from build123d import *

# Parameters (mm, degrees)
BOX008_W                  = 10
BOX008_H                  = 10
BOX008_DEPTH              = 10
BOX008_PLACEMENT_ANGLE    = 45
BOX010_W                  = 10
BOX010_H                  = 10
BOX010_DEPTH              = 10
BOX010_PLACEMENT_ANGLE    = 45
BOX011_W                  = 10
BOX011_H                  = 10
BOX011_DEPTH              = 10
BOX011_PLACEMENT_ANGLE    = 45
BOX009_W                  = 10
BOX009_H                  = 10
BOX009_DEPTH              = 10
BOX009_PLACEMENT_ANGLE    = 45
CYLINDER002_R             = 20
CYLINDER002_DEPTH         = 105
CYLINDER003_R             = 20
CYLINDER003_DEPTH         = 105
CYLINDER001_R             = 3
CYLINDER001_DEPTH         = 105
BOX004_W                  = 105
BOX004_H                  = 105
BOX004_DEPTH              = 3
BOX004_PLACEMENT_ANGLE    = 60
BOX005_W                  = 105
BOX005_H                  = 105
BOX005_DEPTH              = 3
BOX005_PLACEMENT_ANGLE    = 60
BOX006_W                  = 105
BOX006_H                  = 105
BOX006_DEPTH              = 3
FUSION001_PLACEMENT_ANGLE = 90
CYLINDER_R                = 3
CYLINDER_DEPTH            = 105
BOX003_W                  = 105
BOX003_H                  = 105
BOX003_DEPTH              = 3
BOX003_PLACEMENT_ANGLE    = 300
BOX002_W                  = 105
BOX002_H                  = 105
BOX002_DEPTH              = 3
BOX002_PLACEMENT_ANGLE    = 60
BOX001_W                  = 105
BOX001_H                  = 105
BOX001_DEPTH              = 3
CYLINDER005_R             = 2
CYLINDER005_DEPTH         = 10
CYLINDER004_R             = 2
CYLINDER004_DEPTH         = 10
BOX007_W                  = 4
BOX007_H                  = 4
BOX007_DEPTH              = 10
FUSION004_PLACEMENT_ANGLE = 90
BOX_W                     = 12
BOX_H                     = 4
BOX_DEPTH                 = 12
FILLET_R                  = 3


with BuildPart() as cube008:
    # Box008 → Box008 (new body)
    with BuildSketch(Plane.XY):
        with Locations((5, 5)):
            Rectangle(BOX008_W, BOX008_H)
    extrude(amount=BOX008_DEPTH)


with BuildPart() as cube008_1:
    # Box008 placement: moved
    add(cube008.part.moved(Location((-3, -11, 0))).rotate(Axis((-3, -11, 0), (0, 0, 1)), BOX008_PLACEMENT_ANGLE))


with BuildPart() as cube010:
    # Box010 → Box010 (new body)
    with BuildSketch(Plane.XY):
        with Locations((5, 5)):
            Rectangle(BOX010_W, BOX010_H)
    extrude(amount=BOX010_DEPTH)


with BuildPart() as cube010_1:
    # Box010 placement: moved
    add(cube010.part.moved(Location((108.2, -11, 0))).rotate(Axis((108.2, -11, 0), (0, 0, 1)), BOX010_PLACEMENT_ANGLE))


with BuildPart() as cube011:
    # Box011 → Box011 (new body)
    with BuildSketch(Plane.XY):
        with Locations((5, 5)):
            Rectangle(BOX011_W, BOX011_H)
    extrude(amount=BOX011_DEPTH)


with BuildPart() as cube011_1:
    # Box011 placement: moved
    add(cube011.part.moved(Location((108.2, 101.8, 0))).rotate(Axis((108.2, 101.8, 0), (0, 0, 1)), BOX011_PLACEMENT_ANGLE))


with BuildPart() as fusion005:
    # Box009 → Box009 (new body)
    with BuildSketch(Plane.XY):
        with Locations((5, 5)):
            Rectangle(BOX009_W, BOX009_H)
    extrude(amount=BOX009_DEPTH)


with BuildPart() as fusion005_1:
    # Box009 placement: moved
    add(fusion005.part.moved(Location((-3, 102, 0))).rotate(Axis((-3, 102, 0), (0, 0, 1)), BOX009_PLACEMENT_ANGLE))

    # Fusion005: union Cube008, Cube010, Cube011
    add(cube008_1.part)
    add(cube010_1.part)
    add(cube011_1.part)


with BuildPart() as cylinder002:
    # Cylinder002 → Cylinder002 (new body)
    with BuildSketch(Plane(origin=(52.5, 105, 40), x_dir=(1, 0, 0), z_dir=(0, -1, 0))):
        Circle(CYLINDER002_R)
    extrude(amount=CYLINDER002_DEPTH)


with BuildPart() as fusion003:
    # Cylinder003 → Cylinder003 (new body)
    with BuildSketch(Plane(origin=(0, 52.5, 40), x_dir=(0, 0, -1), z_dir=(1, 0, 0))):
        Circle(CYLINDER003_R)
    extrude(amount=CYLINDER003_DEPTH)

    # Fusion003: union Cylinder002
    add(cylinder002.part)


with BuildPart() as cylinder001:
    # Cylinder001 → Cylinder001 (new body)
    with BuildSketch(Plane(origin=(0, 52.5, 92), x_dir=(0, 0, -1), z_dir=(1, 0, 0))):
        Circle(CYLINDER001_R)
    extrude(amount=CYLINDER001_DEPTH)


with BuildPart() as cube004:
    # Box004 → Box004 (new body)
    with BuildSketch(Plane.XY):
        with Locations((52.5, 52.5)):
            Rectangle(BOX004_W, BOX004_H)
    extrude(amount=BOX004_DEPTH)


with BuildPart() as cube004_1:
    # Box004 placement: moved
    add(cube004.part.moved(Location((0, 52.4, 91))).rotate(Axis((0, 52.4, 91), (-1, 0, 0)), BOX004_PLACEMENT_ANGLE))


with BuildPart() as cube005:
    # Box005 → Box005 (new body)
    with BuildSketch(Plane.XY):
        with Locations((52.5, 52.5)):
            Rectangle(BOX005_W, BOX005_H)
    extrude(amount=BOX005_DEPTH)


with BuildPart() as cube005_1:
    # Box005 placement: moved
    add(cube005.part.rotate(Axis((0, 0, 0), (1, 0, 0)), BOX005_PLACEMENT_ANGLE))


with BuildPart() as fusion001:
    # Box006 → Box006 (new body)
    with BuildSketch(Plane.XY):
        with Locations((52.5, 52.5)):
            Rectangle(BOX006_W, BOX006_H)
    extrude(amount=BOX006_DEPTH)

    # Fusion001: union Cylinder001, Cube004, Cube005
    add(cylinder001.part)
    add(cube004_1.part)
    add(cube005_1.part)


with BuildPart() as fusion001_1:
    # Fusion001 placement: moved
    add(fusion001.part.moved(Location((105, 0, 0))).rotate(Axis((105, 0, 0), (0, 0, 1)), FUSION001_PLACEMENT_ANGLE))


with BuildPart() as cylinder:
    # Cylinder → Cylinder (new body)
    with BuildSketch(Plane(origin=(0, 52.5, 92), x_dir=(0, 0, -1), z_dir=(1, 0, 0))):
        Circle(CYLINDER_R)
    extrude(amount=CYLINDER_DEPTH)


with BuildPart() as cube003:
    # Box003 → Box003 (new body)
    with BuildSketch(Plane.XY):
        with Locations((52.5, 52.5)):
            Rectangle(BOX003_W, BOX003_H)
    extrude(amount=BOX003_DEPTH)


with BuildPart() as cube003_1:
    # Box003 placement: moved
    add(cube003.part.moved(Location((0, 52.4, 91))).rotate(Axis((0, 52.4, 91), (1, 0, 0)), BOX003_PLACEMENT_ANGLE))


with BuildPart() as cube002:
    # Box002 → Box002 (new body)
    with BuildSketch(Plane.XY):
        with Locations((52.5, 52.5)):
            Rectangle(BOX002_W, BOX002_H)
    extrude(amount=BOX002_DEPTH)


with BuildPart() as cube002_1:
    # Box002 placement: moved
    add(cube002.part.rotate(Axis((0, 0, 0), (1, 0, 0)), BOX002_PLACEMENT_ANGLE))


with BuildPart() as cut002:
    # Box001 → Box001 (new body)
    with BuildSketch(Plane.XY):
        with Locations((52.5, 52.5)):
            Rectangle(BOX001_W, BOX001_H)
    extrude(amount=BOX001_DEPTH)

    # Fusion: union Cylinder, Cube003, Cube002
    add(cylinder.part)
    add(cube003_1.part)
    add(cube002_1.part)

    # Fusion002: union Fusion001
    add(fusion001_1.part)

    # Cut: cut Fusion003
    add(fusion003.part, mode=Mode.SUBTRACT)

    # Cut002: cut Fusion005
    add(fusion005_1.part, mode=Mode.SUBTRACT)


with BuildPart() as cylinder005:
    # Cylinder005 → Cylinder005 (new body)
    with BuildSketch(Plane.XY):
        Circle(CYLINDER005_R)
    extrude(amount=CYLINDER005_DEPTH)


with BuildPart() as cylinder004:
    # Cylinder004 → Cylinder004 (new body)
    with BuildSketch(Plane(origin=(4, 0, 0), x_dir=(1, 0, 0), z_dir=(0, 0, 1))):
        Circle(CYLINDER004_R)
    extrude(amount=CYLINDER004_DEPTH)


with BuildPart() as fusion004:
    # Box007 → Box007 (new body)
    with BuildSketch(Plane(origin=(0, -2, 0), x_dir=(1, 0, 0), z_dir=(0, 0, 1))):
        with Locations((2, 2)):
            Rectangle(BOX007_W, BOX007_H)
    extrude(amount=BOX007_DEPTH)

    # Fusion004: union Cylinder005, Cylinder004
    add(cylinder005.part)
    add(cylinder004.part)


with BuildPart() as fusion004_1:
    # Fusion004 placement: moved
    add(fusion004.part.moved(Location((50.5, 57, 99))).rotate(Axis((50.5, 57, 99), (1, 0, 0)), FUSION004_PLACEMENT_ANGLE))


with BuildPart() as obj1:
    # Box → Box (new body)
    with BuildSketch(Plane(origin=(46.5, 50.5, 91), x_dir=(1, 0, 0), z_dir=(0, 0, 1))):
        with Locations((6, 2)):
            Rectangle(BOX_W, BOX_H)
    extrude(amount=BOX_DEPTH)

    # Fillet
    fillet_edges = [obj1.edges().sort_by_distance(p)[0] for p in [
        (46.5, 52.5, 103),
        (58.5, 52.5, 103),
    ]]
    fillet(fillet_edges, radius=FILLET_R)

    # Cut001: cut Fusion004
    add(fusion004_1.part, mode=Mode.SUBTRACT)

    # Fusion006: union Cut002
    add(cut002.part)


solid = obj1.part
For this review, take the finished solid that the model builds, in its own axes (mm). A direction names the side the tool comes from. Round coordinates to 2 decimals unless told otherwise and drop trailing zeros. Loops run counter-clockwise (first coordinate to the right, second up) from the corner with the lowest first, then second, coordinate; pieces in that order, holes last. Notation, with made-up numbers: (37, -21) - (90, -21) arc R13 ccw to (90, -9) - close; hole circle Ø11 at (81.5, -35). An arc over 180 degrees is marked (long way). Use one line per item in the form item = value.
Item 1: Tool access review of faces 5 (the flat face through (52.33, 7.83, 19.56)), 6 (the flat face through (11.81, 44.72, 20.35)), 7 (the flat face through (52, 53, 101)): name each direction out of +Z, -Z, +X, -X, +Y, -Y from which nothing blocks a thin tool from reaching the whole face with its end or side.
Answers:
face_5 = -Y
face_6 = none
face_7 = +Y, -Y
Item 2: Clearance check with flat-ended pins moving along their axes: P1, Ø24, axis at y = 52.5, z = 40, coming from the +X side; P2, Ø12, axis at x = 38, z = 35.5, coming from the -Y side; P3, Ø3, axis at y = 53.5, z = 96, coming from the -X side; P4, Ø12, axis at x = 10.5, y = 91, coming from the -Z side. State where each tip first meets the part, or that it passes through.
Answers:
P1 = through
P2 = 14.03
P3 = 0
P4 = 0
Item 3: For line 1 (Z direction, x = 27, y = 52.5); line 2 (Y direction, x = 20, z = 40); line 3 (Z direction, x = 52, y = 62), list the stretches that pass through material, from the lowest coordinate up.
Answers:
line_1 = 0 to 3, 89 to 95
line_2 = 0 to 32.5, 72.5 to 105
line_3 = 0 to 3, 74.37 to 80.37, 89.04 to 94.96
Item 4: Consider section A-A on y = 93. Write out the cut boundary in (x, z), then the cut area to 3 significant figures.
Answers:
outline = (-2.5, 1.57) - (0, 0.13) - (0, 0) - (105, 0) - (107.6, 1.5) - (96.53, 20.68) - (105, 20.68) - (105, 26.68) - (93.06, 26.68) - (55.49, 91.75) arc R3 ccw (long way) to (49.52, 91.66) - (12, 26.68) - (0, 26.68) - (0, 20.68) - (8.54, 20.68) - close; hole (1.79, 3) - (103.27, 3) - (93.06, 20.68) - (57.67, 20.68) arc R20 ccw to (67.42, 26.68) - (89.6, 26.68) - (53.51, 89.18) arc R3 cw to (51.54, 89.16) - (15.46, 26.68) - (37.58, 26.68) arc R20 ccw to (47.33, 20.68) - (12, 20.68) - close
area = 1,410 mm^2
Item 5: Consider section C-C on x = 84.5. Write out the cut boundary in (y, z), then the cut area to 3 significant figures.
Answers:
outline = (-2.6, 1.5) - (0, 0) - (105, 0) - (105, 0.13) - (107.5, 1.57) - (87.9, 35.51) - (105, 35.51) - (105, 41.51) - (84.44, 41.51) - (55.48, 91.66) arc R3 ccw (long way) to (49.51, 91.75) - (20.5, 41.51) - (0, 41.51) - (0, 35.51) - (17.04, 35.51) - close; hole (1.73, 3) - (103.21, 3) - (84.44, 35.51) - (71.99, 35.51) arc R20 ccw to (72.44, 41.51) - (80.97, 41.51) - (53.46, 89.16) arc R3 cw to (51.49, 89.18) - (23.96, 41.51) - (32.56, 41.51) arc R20 ccw to (33.01, 35.51) - (20.5, 35.51) - close
area = 1,310 mm^2
Item 6: Mouldability with a two-part tool opening along X and no side actions: class faces 1 (the flat face through (18.9, 30.6, 59)), 2 (the flat face through (29.955, 18.887, 57.778)), 3 (the flat face through (37.864, 13.001, 65.477)), 4 (the flat face through (105, 105, 2)) as +X half, -X half, draft (parallel to the pull), parting line (faces both ways), or undercut.
Answers:
face_1 = draft
face_2 = -X half
face_3 = undercut
face_4 = +X half
Item 7: Consider section D-D on z = 47.5. State how many separate pieces and enclosed holes the cut face has, then the cut area to 3 significant figures.
Answers:
separate_pieces = 4
enclosed_holes = 0
area = 893 mm^2
